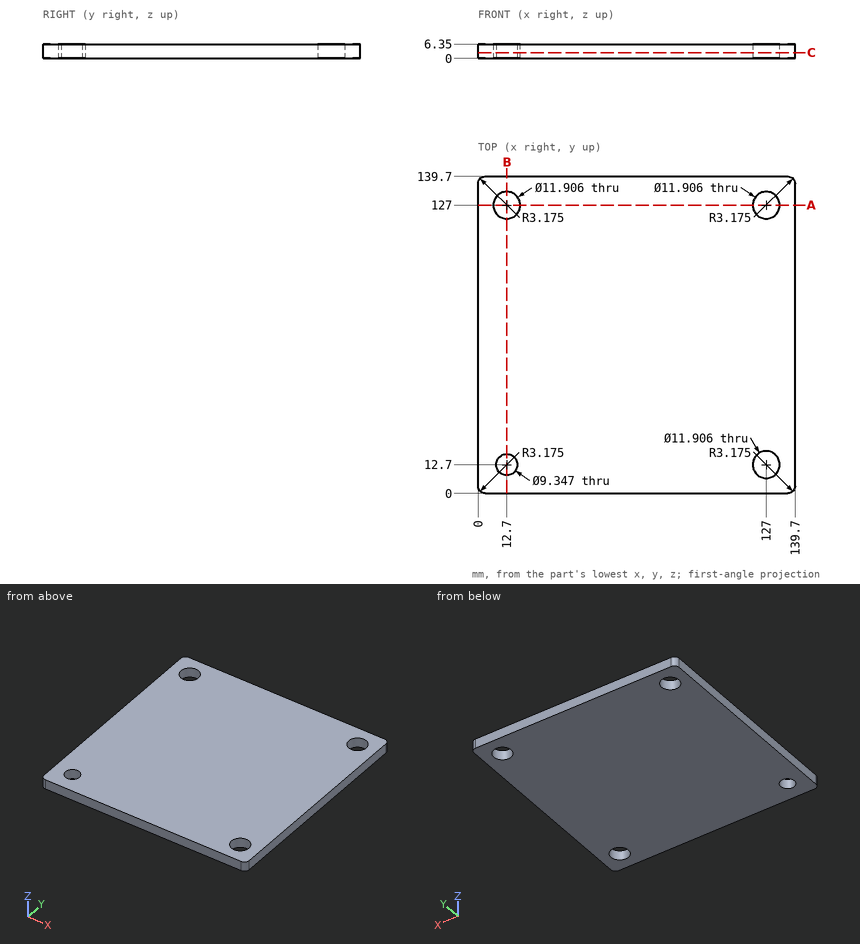
Design review of the part shown in the three views and the two pictorial views. Dimensions are in mm from the part's minimum x, y and z. Round coordinates to 2 decimals unless told otherwise and drop trailing zeros. Write each loop counter-clockwise with the first axis right and the second up, starting at its lowest first coordinate (ties: lowest second). Pieces come first, ordered by that corner, then holes.
Item 1: For probe 1 along Y at (x, z) = (12.7, 4); probe 2 along Y at (x, z) = (127, 2); probe 3 along X at (y, z) = (11.5, 5.5), list the stretches that pass through material, from the lowest coordinate up.
Item 2: Clearance check with a flat-ended pin moving along its axis: pin 1 Ø10.5 at (x, y) = (12.7, 127) entering from -Z (1 decimal). State where the tip first meets the part, or that it passes through.
Item 3: We need section B-B on x = 12.7. Write out the cut boundary in (y, z), and give its area (3 significant figures).
Item 4: We need section C-C on z = 2.5. State how many separate pieces and enclosed holes the cut face has, and give its area (3 significant figures).
Item 5: We need section A-A on y = 127. Write out the cut boundary in (x, z), and give its area (3 significant figures).
Returned:
1. probe 1: y = 0 to 8.03, 17.37 to 121.05, 132.95 to 139.7
1. probe 2: y = 0 to 6.75, 18.65 to 121.05, 132.95 to 139.7
1. probe 3: x = 0 to 8.18, 17.22 to 121.17, 132.83 to 139.7
2. pin 1: passes through
3. outline: (0, 0) - (8.03, 0) - (8.03, 6.35) - (0, 6.35) - close; (17.37, 0) - (121.05, 0) - (121.05, 6.35) - (17.37, 6.35) - close; (132.95, 0) - (139.7, 0) - (139.7, 6.35) - (132.95, 6.35) - close
3. area: 752 mm2
4. separate pieces: 1
4. enclosed holes: 4
4. area: 19,100 mm2
5. outline: (0, 0) - (6.75, 0) - (6.75, 6.35) - (0, 6.35) - close; (18.65, 0) - (121.05, 0) - (121.05, 6.35) - (18.65, 6.35) - close; (132.95, 0) - (139.7, 0) - (139.7, 6.35) - (132.95, 6.35) - close
5. area: 736 mm2
